Could you check a few things on this drawing? It's one solid part, dimensions in mm from its lowest x, y, z. Coordinates: 2 decimals unless noted, no trailing zeros. Write each loop counter-clockwise with the first axis right and the second up, starting at its lowest first coordinate (ties: lowest second). Pieces come first, ordered by that corner, then holes.
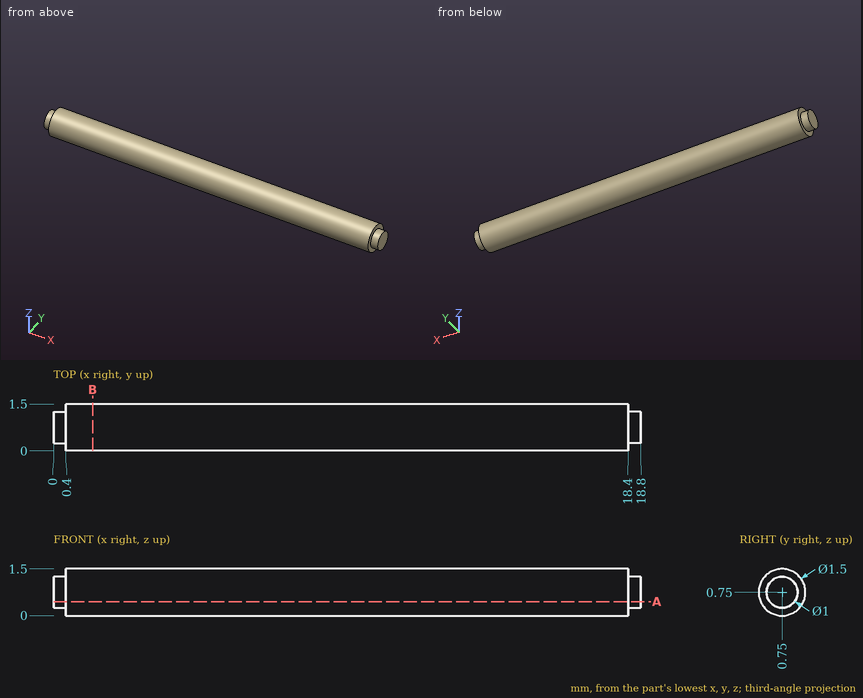
1) I need wall thicknesses on probe 1 along X at (y, z) = (0.3, 0.45); probe 2 along Z at (x, y) = (10.75, 0.8). Which ranges of each line are inside material? Lowest first, please.
Values follow:
probe 1: x = 0.4 to 18.4
probe 2: z = 0 to 1.5
2) Imagine slicing it at A-A on z = 0.45. Please give me the cut outline in (x, y), then the cut area to 3 significant figures.
Values follow:
outline: (0, 0.35) - (0.4, 0.35) - (0.4, 0.06) - (18.4, 0.06) - (18.4, 0.35) - (18.8, 0.35) - (18.8, 1.15) - (18.4, 1.15) - (18.4, 1.44) - (0.4, 1.44) - (0.4, 1.15) - (0, 1.15) - close
area: 25.4 mm2
3) Imagine slicing it at B-B on x = 1.25. Please give me the cut outline in (y, z), then the cut area to 3 significant figures.
Values follow:
outline: circle Ø1.5 at (0.75, 0.75)
area: 1.77 mm2
